Read the model definition and answer for the solid it produces. Units are mm, in the model's axes. Face numbers are marked on the shaded views. Coordinates: 2 decimals unless noted, no trailing zeros. Loops run counter-clockwise (first coordinate to the right, second up) from the corner with the lowest first, then second, coordinate; pieces in that order, holes last. Notation, with made-up numbers: (45.5, -33) -> (61.5, -33) arc R19 cw to (61.5, -19) -> close; hole circle Ø5 at (88, -28). An arc over 180 degrees is marked (long way). Answer as a JSON object with one key per item and string values. Group by question number.
Q1. Each of these flat-tipped pins is pushed along its axis until it touches: P1, Ø2, axis at x = 13.5, z = -0.5, coming from the +Y side; P2, Ø1, axis at y = 5, z = 2, coming from the -X side; P3, Ø2.5, axis at x = 31, z = 0, coming from the +Y side. Where does it stop, or does it pass through?
Q2. Straight lines are drawn through the part: line 1 along X through (y, z) = (8.75, 0); line 2 along Y through (x, z) = (27.5, -1.25); line 3 along X through (y, z) = (6.75, 1.75). For each, find the intervals that lie inside material, in ascending order. Write a range as [from, to].
Q3. The part is cut by section C-C on x = 20.5. Write down the section's boundary in (y, z), and give its area (3 significant figures).
Q4. Determine the mould class of the marked faces 1, 2 and 3 for opening direction X: released by +X, released by -X, zero draft, split by the parting line, or undercut.
Q5. The part is cut by section A-A on y = 7.25. Write down the section's boundary in (x, z).
Q6. The part is cut by section B-B on x = 30. Write down the section's boundary in (y, z), and give its area (3 significant figures).
from build123d import *

# Parameters (mm, degrees)
SKETCH1_W           = 37
SKETCH1_H           = 31
SKETCH1_R           = 1.5
BOSS_EXTRUDE1_DEPTH = 2
SKETCH2_R           = 3
SKETCH2_R_2         = 1.5
BOSS_EXTRUDE2_DEPTH = 20
SKETCH3_W           = 37
SKETCH3_H           = 24
CUT_EXTRUDE1_DEPTH  = 50.2341345


with BuildPart() as part:
    # Sketch1 → Boss-Extrude1 (new body)
    with BuildSketch(Plane(origin=(0, 0, 0), x_dir=(1, 0, 0), z_dir=(0, 1, 0))):
        with Locations((15.5, 12.5)):
            Rectangle(SKETCH1_W, SKETCH1_H)
        with Locations(Location((0, 25, 0), (0, 0, 270))):
            Circle(SKETCH1_R, mode=Mode.SUBTRACT)
        with Locations(Location((31, 25, 0), (0, 0, 270))):
            Circle(SKETCH1_R, mode=Mode.SUBTRACT)
        with Locations(Location((31, 0, 0), (0, 0, 270))):
            Circle(SKETCH1_R, mode=Mode.SUBTRACT)
        with Locations(Location((0, 0, 0), (0, 0, 270))):
            Circle(SKETCH1_R, mode=Mode.SUBTRACT)
    extrude(amount=BOSS_EXTRUDE1_DEPTH)

    # Sketch2 → Boss-Extrude2 (add)
    # profile 1 of 4: a face of its own
    with BuildSketch(Plane(origin=(0, 2, 0), x_dir=(1, 0, 0), z_dir=(0, 1, 0))):
        with Locations(Location((0, 25, 0), (0, 0, 90))):
            Circle(SKETCH2_R)
        with Locations(Location((0, 25, 0), (0, 0, 270))):
            Circle(SKETCH2_R_2, mode=Mode.SUBTRACT)
    # profile 2 of 4: a face of its own
    with BuildSketch(Plane(origin=(0, 2, 0), x_dir=(1, 0, 0), z_dir=(0, 1, 0))):
        with Locations(Location((31, 25, 0), (0, 0, 90))):
            Circle(SKETCH2_R)
        with Locations(Location((31, 25, 0), (0, 0, 270))):
            Circle(SKETCH2_R_2, mode=Mode.SUBTRACT)
    # profile 3 of 4: a face of its own
    with BuildSketch(Plane(origin=(0, 2, 0), x_dir=(1, 0, 0), z_dir=(0, 1, 0))):
        with Locations(Location((31, 0, 0), (0, 0, 270))):
            Circle(SKETCH2_R)
        with Locations(Location((31, 0, 0), (0, 0, 270))):
            Circle(SKETCH2_R_2, mode=Mode.SUBTRACT)
    # profile 4 of 4: a face of its own
    with BuildSketch(Plane(origin=(0, 2, 0), x_dir=(1, 0, 0), z_dir=(0, 1, 0))):
        with Locations(Location((0, 0, 0), (0, 0, 270))):
            Circle(SKETCH2_R)
        with Locations(Location((0, 0, 0), (0, 0, 270))):
            Circle(SKETCH2_R_2, mode=Mode.SUBTRACT)
    extrude(amount=BOSS_EXTRUDE2_DEPTH)

    # Sketch3 → Cut-Extrude1 (cut, through all)
    with BuildSketch(Plane.XZ):
        with Locations((15.5, -16)):
            Rectangle(SKETCH3_W, SKETCH3_H)
    extrude(amount=-CUT_EXTRUDE1_DEPTH, mode=Mode.SUBTRACT)


solid = part.part
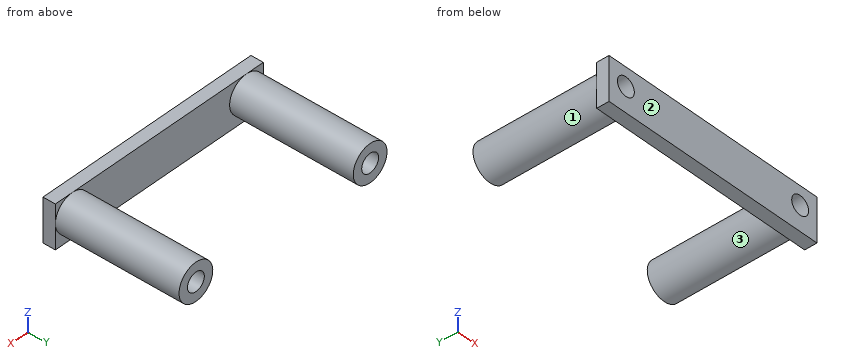
Final values:
{
 "1": {"P1": "stops at y = 2", "P2": "stops at x = -2.6", "P3": "passes through"},
 "2": {"line 1": "x = [-3, -1.5], [1.5, 3], [28, 29.5], [32.5, 34]", "line 2": "y = [0, 2]", "line 3": "x = [-2.44, 2.44], [28.56, 33.44]"},
 "3": {"outline": "(0, -4) -> (2, -4) -> (2, 3) -> (0, 3) -> close", "area": "14.0 mm2"},
 "4": {"face 1": "undercut", "face 2": "zero draft", "face 3": "undercut"},
 "5": {"outline": "circle Ø6 at (0, 0); circle Ø6 at (31, 0); hole circle Ø3 at (0, 0); hole circle Ø3 at (31, 0)"},
 "6": {"outline": "(0, -4) -> (2, -4) -> (2, -2.83) -> (22, -2.83) -> (22, -1.12) -> (0, -1.12) -> close; (0, 1.12) -> (22, 1.12) -> (22, 2.83) -> (2, 2.83) -> (2, 3) -> (0, 3) -> close", "area": "77.9 mm2"}
}
